Source: CAD feature listing. Evaluate the final solid. Frame: model axes, mm. A direction names the side the tool comes from. Give positions to 0.01 mm unless a question says otherwise; leave off trailing zeros. Loops run counter-clockwise (first coordinate to the right, second up) from the corner with the lowest first, then second, coordinate; pieces in that order, holes last. Notation, with made-up numbers: (29.5, 32.5) -> (38.5, 32.5) arc R7 cw to (38.5, 45.5) -> close; hole circle Ø4 at (68, 71). An arc over 180 degrees is marked (long way). Put each result on its own line as item: value.
```python
from build123d import *


with BuildPart() as part:
    # Sketch1 → Revolve1 (revolve)
    with BuildSketch(Plane.XY, mode=Mode.PRIVATE) as revolve1_sk:
        Polygon((20, 49), (20, 45), (11, 43), (11, 24), (21, 22), (21, 7), (19.765711135, 0), (19, 0), (19, 20), (8, 20), (8, 31), (2, 31), (2, 33), (4, 33), (4, 35.5), (8, 35.5), (8, 47), (18, 47), (18, 51), align=None)
    revolve(revolve1_sk.sketch.rotate(Axis((0, 0, 0), (0, 1, 0)), 90), axis=Axis((0, 0, 0), (0, 1, 0)))


solid = part.part
```
(1) Line query: probe 1 along X at (y, z) = (48, 0); probe 2 along X at (y, z) = (34, 0); probe 3 along Z at (x, y) = (-2.5, 47.5). Output: solid intervals per line, ascending. Write a range as from..to.
Calculated:
probe 1: x = -20..-18, 18..20
probe 2: x = -11..-4, 4..11
probe 3: z = -19.84..-17.83, 17.83..19.84
(2) Reachability of faces 1 (the cylindrical face through (-12.165, 49.028, 13.267)), 2 (the flat face through (2, 31, -2)), 3 (the cylindrical face through (10.74, 33.37, 2.38)) from +Z, -Z, +X, -X, +Y, -Y: full face, straight path, thin tool, end or side. Return the list, or none.
Calculated:
face 1: +Y
face 2: -Y
face 3: none
(3) Section A-A on y = 23. Return loops of the section in (x, z).
Calculated:
outline: circle Ø32 at (0, 0); hole circle Ø16 at (0, 0)
(4) Draft query along X for faces 4 (the cylindrical face through (-0.88, 46.97, 19.98)), 5 (the cylindrical face through (7.81, 25.58, 1.73)), 6 (the flat face through (-16.2, 0, 10.3)). Return one class per face: released by +X, released by -X, zero draft, split by the parting line, or undercut.
Calculated:
face 4: split by the parting line
face 5: undercut
face 6: zero draft
(5) First-contact query: P1, Ø5, axis at x = 2, z = 0, coming from the -Y side; P2, Ø8, axis at x = 8, z = -7.5, coming from the -Y side; P3, Ø8, axis at x = 0.5, z = -2, coming from the +Y side. Flat tips, straight axial feed; report the tip coordinate or a pass-through.
Calculated:
P1: stops at y = 31
P2: stops at y = 20
P3: stops at y = 35.5
